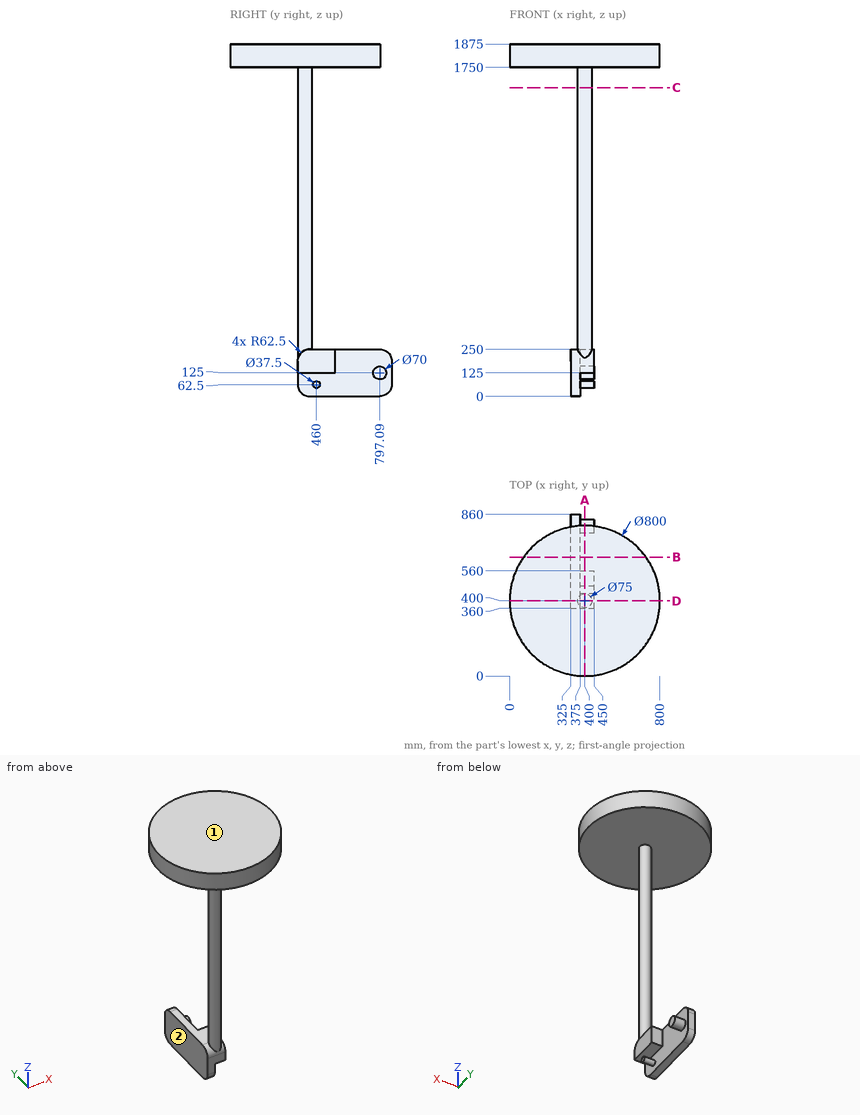
Part print with two shaded views. Sizes in mm from the minimum x, y, z corner. A direction names the side the tool comes from. Round coordinates to 2 decimals unless told otherwise and drop trailing zeros. Order: outer loops, then holes, each group sorted by start corner. A loop starts at its lowest first (then second) coordinate and runs counter-clockwise, first axis right, second up. Notation, with made-up numbers: (73.25, 58.25) - (123.25, 58.25) arc R27 cw to (123.25, 95.25) - close; hole circle Ø6 at (40, 80.25). An arc over 180 degrees is marked (long way). Return JSON: item names as keys, results as strings.
(1) Tool access for the marked faces 1 and 2: list every direction of +Z, -Z, +X, -X, +Y, -Y with a clear straight run to the whole face (end or side of a thin tool).
Answer key:
{"face 1": "+Z, +X, -X, +Y, -Y", "face 2": "-Z, -X, +Y, -Y"}
(2) Cut at C-C (z = 1642.5). Give the cut face in (x, y), then the cut area to 3 significant figures.
Answer key:
{"outline": "circle Ø75 at (400, 400)", "area": "4,420 mm^2"}
(3) Cut at B-B (y = 633). Give the cut face in (x, z).
Answer key:
{"outline": "(74.87, 1750) - (725.13, 1750) - (725.13, 1875) - (74.87, 1875) - close; (325, 0) - (375, 0) - (375, 250) - (325, 250) - close"}
(4) Wall check: probe 1 along Z at (x, y) = (399.5, 581); probe 2 along Z at (x, y) = (437.5, 439.5); probe 3 along X at (y, z) = (544, 1790). Give the ranges that are in metal, low to high. Write a range as from..to.
Answer key:
{"probe 1": "z = 1750..1875", "probe 2": "z = 125..250, 1750..1875", "probe 3": "x = 26.82..773.18"}
(5) Cut at A-A (x = 400). Give the cut face in (y, z).
Answer key:
{"outline": "(0, 1750) - (362.5, 1750) - (362.5, 205) arc R62.5 ccw to (360, 187.5) - (360, 125) - (560, 125) - (560, 250) - (437.5, 250) - (437.5, 1750) - (800, 1750) - (800, 1875) - (0, 1875) - close; circle Ø37.5 at (460, 62.5); circle Ø70 at (797.09, 125)"}
(6) Cut at D-D (y = 400). Give the cut face in (x, z), then the cut area to 3 significant figures.
Answer key:
{"outline": "(0, 1750) - (362.5, 1750) - (362.5, 245.81) - (325, 245.81) - (325, 4.19) - (375, 4.19) - (375, 125) - (450, 125) - (450, 245.81) - (437.5, 245.81) - (437.5, 1750) - (800, 1750) - (800, 1875) - (0, 1875) - close", "area": "234,000 mm^2"}
(7) Pin check, flat tips, straight feed: pin 1 Ø6 at (x, y) = (320, 713.5) entering from -Z; pin 2 Ø22.5 at (x, z) = (417.5, 217.5) entering from +Y. Stop position of each tip, or through.
Answer key:
{"pin 1": "stops at z = 1750", "pin 2": "stops at y = 560"}
